Here's the drawing with two shaded views (mm, measured from the low corner). I have some questions. A direction names the side the tool comes from. Round coordinates to 2 decimals unless told otherwise and drop trailing zeros. Order: outer loops, then holes, each group sorted by start corner. A loop starts at its lowest first (then second) coordinate and runs counter-clockwise, first axis right, second up. Notation, with made-up numbers: M 5.25,-13.75 L 9.25,-13.75 A18 ccw 9.25,-3.75 Z; hole C 59.5,37 d11. An arc over 180 degrees is marked long. One line per question, with ' | ' between items.
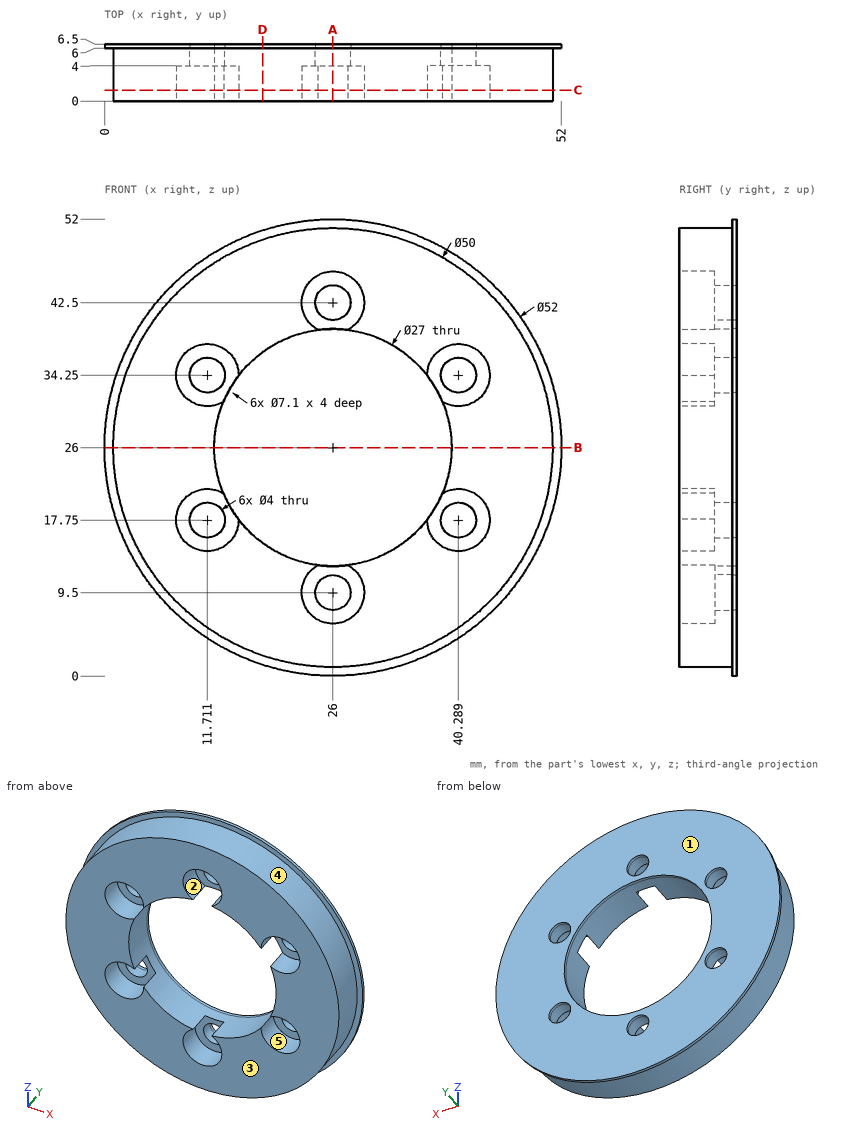
(1) Thinking about a two-plate mould opening in Z: for the marked faces 3, 4 and 5, which applies, released by +Z, released by -Z, zero draft, split by the parting line, or undercut?
Final values:
face 3: zero draft | face 4: split by the parting line | face 5: undercut
(2) Will these pins go through, and if not, where does the flat tip stop? pin 1 Ø3 at (x, y) = (30.5, 1) entering from +Z; pin 2 Ø2 at (x, z) = (27.5, 8) entering from -Y; pin 3 Ø2 at (x, y) = (37.5, 3.5) entering from +Z.
Final values:
pin 1: z = 50.82 | pin 2: y = 4 | pin 3: z = 48.69
(3) If we section it at D-D on x = 18: Please give me the cut outline in (y, z) (1 decimal), plus the area to 3 significant figures.
Final values:
outline: M 0,2.3 L 6,2.3 L 6,1.3 L 6.5,1.3 L 6.5,15.1 L 0,15.1 Z; M 0,36.9 L 6.5,36.9 L 6.5,50.7 L 6,50.7 L 6,49.7 L 0,49.7 Z | area: 168 mm^2
(4) Please list where these lines run through material, in increasing order: probe 1 along Z at (x, y) = (11, 5); probe 2 along X at (y, z) = (5.25, 35) (1 decimal); probe 3 along X at (y, z) = (3, 21) (1 decimal). Write a range as [from, to].
Final values:
probe 1: [6, 15.88], [19.62, 32.38], [36.12, 46] | probe 2: [2.7, 9.9], [13.6, 15.9], [36.1, 38.4], [42.1, 49.3] | probe 3: [1.5, 10.3], [13.1, 13.5], [38.5, 38.9], [41.7, 50.5]
(5) If we section it at C-C on y = 1.25: Please give me the cut outline in (x, z).
Final values:
outline: C 26,26 d50; hole M 13.55,20.79 A3.55 ccw long 15.26,17.82 A13.5 ccw 24.29,12.61 A3.55 ccw long 27.71,12.61 A13.5 ccw 36.74,17.82 A3.55 ccw long 38.45,20.79 A13.5 ccw 38.45,31.21 A3.55 ccw long 36.74,34.18 A13.5 ccw 27.71,39.39 A3.55 ccw long 24.29,39.39 A13.5 ccw 15.26,34.18 A3.55 ccw long 13.55,31.21 A13.5 ccw Z
(6) If we section it at B-B on z = 26: Please give me the cut outline in (x, y).
Final values:
outline: M 0,6 L 1,6 L 1,0 L 12.5,0 L 12.5,6.5 L 0,6.5 Z; M 39.5,0 L 51,0 L 51,6 L 52,6 L 52,6.5 L 39.5,6.5 Z
(7) On a 3-axis mill with a long thin cutter (end or side, diameter ignored), from which of +Z, -Z, +X, -X, +Y, -Y can I reach the whole of each face in a straight line? I mean the marked faces 1 and 2. Say none if no direction works.
Final values:
face 1: +Z, -Z, +X, -X, +Y | face 2: -Y
(8) If we section it at A-A on x = 26: Please give me the cut outline in (y, z).
Final values:
outline: M 0,1 L 6,1 L 6,0 L 6.5,0 L 6.5,7.5 L 4,7.5 L 4,5.95 L 0,5.95 Z; M 0,46.05 L 4,46.05 L 4,44.5 L 6.5,44.5 L 6.5,52 L 6,52 L 6,51 L 0,51 Z; M 4,11.5 L 6.5,11.5 L 6.5,12.5 L 4,12.5 Z; M 4,39.5 L 6.5,39.5 L 6.5,40.5 L 4,40.5 Z
